```python
from build123d import *

# Parameters (mm, degrees)
EXTRUDE_1_DEPTH          = 10
SKETCH_2_R               = 8
CUT_EXTRUDE_1_DEPTH      = 10
EXTRUDE_START            = -1.2
SKETCH_4_R               = 8
EXTRUDE_2_DEPTH          = 1.2
CUT_EXTRUDE_4_DEPTH      = 8.8
EXTRUDE_START_2          = 1.2
EXTRUDE_3_DEPTH          = 7.6
SKETCH_6_W               = 0.8
SKETCH_6_H               = 0.8
CUT_EXTRUDE_5_DEPTH      = 0.8
CUT_EXTRUDE_6_DEPTH      = 1.2
SKETCH_8_W               = 1.6
SKETCH_8_H               = 0.8
EXTRUDE_4_DEPTH          = 0.8
HOLE_WIZARD_M2_5_2_D     = 2.05
HOLE_WIZARD_M2_5_2_DEPTH = 10
HOLE_WIZARD_M2_5_2_TIP   = 0.615882135


# Read off the part's stored shape, not the designer's step: 填料-伸長3
with BuildPart() as part:
    # 草圖1 → 填料-伸長1 (new body)
    with BuildSketch(Plane(origin=(0, 0, 0), x_dir=(1, 0, 0), z_dir=(0, 1, 0))):
        with BuildLine():
            ThreePointArc((0, -20), (-5.176380902, -19.318516526), (-10, -17.320508076))
            Line((-10, -17.320508076), (-10, -69.320508076))
            Line((-10, -69.320508076), (10, -69.320508076))
            Line((10, -69.320508076), (10, -17.320508076))
            ThreePointArc((10, -17.320508076), (5.176380902, -19.318516526), (0, -20))
        make_face()
    extrude(amount=EXTRUDE_1_DEPTH)

    # 草圖2 → 除料-伸長1 (cut)
    with BuildSketch(Plane(origin=(0, 10, 0), x_dir=(1, 0, 0), z_dir=(0, 1, 0))):
        with Locations(Location((0, -59.320508076, 0), (0, 0, 270))):
            Circle(SKETCH_2_R)
    extrude(amount=-CUT_EXTRUDE_1_DEPTH, mode=Mode.SUBTRACT)

    # 草圖4 → 填料-伸長2 (add)
    with BuildSketch(Plane.XZ.offset(EXTRUDE_START)):
        with Locations(Location((0, 59.320508076, 0), (0, 0, 90))):
            Circle(SKETCH_4_R)
    extrude(amount=EXTRUDE_2_DEPTH)

    # 草圖5 → 除料-伸長4 (cut)
    with BuildSketch(Plane(origin=(0, 10, 0), x_dir=(1, 0, 0), z_dir=(0, 1, 0))):
        with BuildLine():
            Line((-8, -39.320508076), (-8, -59.320508076))
            ThreePointArc((-8, -59.320508076), (0, -51.320508076), (8, -59.320508076))
            Line((8, -59.320508076), (8, -39.320508076))
            Line((8, -39.320508076), (-8, -39.320508076))
        make_face()
    extrude(amount=-CUT_EXTRUDE_4_DEPTH, mode=Mode.SUBTRACT)

    # 填料-伸長3 outline → 填料-伸長3 (add)
    with BuildSketch(Plane(origin=(0, 0, 0), x_dir=(1, 0, 0), z_dir=(0, 1, 0)).offset(EXTRUDE_START_2)):
        with BuildLine():
            Line((-8, -39.320508076), (-8, -59.320508076))
            ThreePointArc((-8, -59.320508076), (0, -67.320508076), (8, -59.320508076))
            Line((8, -59.320508076), (8, -39.320508076))
            Line((8, -39.320508076), (-8, -39.320508076))
        make_face()
        with BuildLine():
            ThreePointArc((7.2, -59.320508076), (0, -66.520508076), (-7.2, -59.320508076))
            Line((-7.2, -59.320508076), (-7.2, -40.120508076))
            Line((-7.2, -40.120508076), (7.2, -40.120508076))
            Line((7.2, -40.120508076), (7.2, -59.320508076))
        make_face(mode=Mode.SUBTRACT)
    extrude(amount=EXTRUDE_3_DEPTH)

    # 草圖6 → 除料-伸長5 (cut)
    with BuildSketch(Plane(origin=(0, 10, 0), x_dir=(1, 0, 0), z_dir=(0, 1, 0))):
        with Locations((0.4, -38.920508076)):
            Rectangle(SKETCH_6_W, SKETCH_6_H)
        with Locations((-0.4, -38.920508076)):
            Rectangle(SKETCH_6_W, SKETCH_6_H)
    extrude(amount=-CUT_EXTRUDE_5_DEPTH, mode=Mode.SUBTRACT)

    # 草圖7 → 除料-伸長6 (cut)
    with BuildSketch(Plane.XZ):
        with BuildLine():
            Line((10, 69.320508076), (10, 17.320508076))
            ThreePointArc((10, 17.320508076), (0, 20), (-10, 17.320508076))
            Line((-10, 17.320508076), (-10, 69.320508076))
            Line((-10, 69.320508076), (10, 69.320508076))
        make_face()
    extrude(amount=-CUT_EXTRUDE_6_DEPTH, mode=Mode.SUBTRACT)

    # 草圖8 → 填料-伸長4 (add)
    with BuildSketch(Plane(origin=(0, 10, 0), x_dir=(1, 0, 0), z_dir=(0, 1, 0))):
        with Locations((0, -38.920508076)):
            Rectangle(SKETCH_8_W, SKETCH_8_H)
    extrude(amount=-EXTRUDE_4_DEPTH)

    # M2.5  螺絲攻的螺孔鑽2
    with Locations(Plane(origin=(-10, 7.214577241, 60), x_dir=(0, 0, -1), z_dir=(-1, 0, 0))):
        with Locations((0, 0)):
            Hole(HOLE_WIZARD_M2_5_2_D / 2, depth=HOLE_WIZARD_M2_5_2_DEPTH)
            with Locations((0, 0, -(HOLE_WIZARD_M2_5_2_DEPTH + HOLE_WIZARD_M2_5_2_TIP / 2))):  # 118° drill point
                Cone(0, HOLE_WIZARD_M2_5_2_D / 2, HOLE_WIZARD_M2_5_2_TIP, mode=Mode.SUBTRACT)


solid = part.part
```
Design review of the part built by this model. Coordinates are the model's own, in mm. A direction names the side the tool comes from. Coordinates: 2 decimals unless noted, no trailing zeros. Order: outer loops, then holes, each group sorted by start corner. A loop starts at its lowest first (then second) coordinate and runs counter-clockwise, first axis right, second up. Notation, with made-up numbers: (14, 45.25) - (45, 45.25) arc R31 cw to (45, 81.25) - close; hole circle Ø4 at (-7.75, 17.25). An arc over 180 degrees is marked (long way). One line per question, with ' | ' between items.
Q1. To check wall thickness, follow line 1 along Y through (x, z) = (-8.05, 60); line 2 along Z through (x, y) = (-0.25, 6); line 3 along X through (y, z) = (7.5, 49). State the ranges of each line that lie inside material, in increasing order.
Answer key:
line 1: y = 1.2 to 6.19, 8.24 to 10 | line 2: z = 20 to 40.12, 66.52 to 69.32 | line 3: x = -10 to -7.2, 7.2 to 10
Q2. Consider section A-A, the plane z = 58.5. Give the boundary of the cut face in (x, y), then the cut area to 3 significant figures.
Answer key:
outline: (-10, 1.2) - (-7.2, 1.2) - (-7.2, 8.8) - (-8, 8.8) - (-8, 10) - (-10, 10) - close; (7.2, 1.2) - (10, 1.2) - (10, 10) - (8, 10) - (8, 8.8) - (7.2, 8.8) - close | area: 47.4 mm2
Q3. Consider section C-C, the plane x = 0.75. Give the boundary of the cut face in (y, z).
Answer key:
outline: (1.2, 19.99) - (10, 19.99) - (10, 39.32) - (8.8, 39.32) - (8.8, 40.12) - (1.2, 40.12) - close; (1.2, 66.48) - (8.8, 66.48) - (8.8, 67.29) - (10, 67.29) - (10, 69.32) - (1.2, 69.32) - close
Q4. Consider section B-B, the plane y = 2. Give the boundary of the cut face in (x, z).
Answer key:
outline: (-10, 17.32) arc R20 cw to (10, 17.32) - (10, 69.32) - (-10, 69.32) - close; hole (-7.2, 40.12) - (7.2, 40.12) - (7.2, 59.32) arc R7.2 ccw to (-7.2, 59.32) - close
Q5. The part is to be moulded in two halves that separate along Z. For faces 1 (the flat face through (0, 1.2, 38)), 2 (the flat face through (8, 9, 49)), 3 (the flat face through (0, 6, 69.321)), say which applies: +Z half, -Z half, draft (parallel to the pull), parting line (faces both ways), or undercut.
Answer key:
face 1: draft | face 2: undercut | face 3: +Z half
Q6. Clearance check with flat-ended pins moving along their axes: pin 1 Ø1.8 at (y, z) = (7.21, 60) entering from -X; pin 2 Ø1.5 at (x, z) = (5, 46) entering from -Y. State where each tip first meets the part, or that it passes through.
Answer key:
pin 1: stops at x = 7.02 | pin 2: passes through
Q7. For faces 4 (the flat face through (7.2, 5, 50)), 5 (the flat face through (7.7, 8.8, 52.2)), 6 (the cylindrical face through (-8.48, 6.91, 60.98)), 7 (the flat face through (10, 6, 44)), list the 3-axis set-ups (+Z, -Z, +X, -X, +Y, -Y) from which the entire face can be reached by the end or side of a thin tool; tool diameter is ignored.
Answer key:
face 4: +Y, -Y | face 5: +Y | face 6: -X | face 7: +Z, -Z, +X, +Y, -Y
